from build123d import *

# Parameters (mm, degrees)
F0_R     = 9
F1_DEPTH = 19.3
F2_R     = 1
F3_R     = 4.68
F4_DEPTH = 10
F5_R     = 4
F6_DEPTH = 25


with BuildPart() as f1:
    # F0 (on Front) → F1 (new body)
    with BuildSketch(Plane.XZ):
        with BuildLine():
            ThreePointArc((-15.21127, 25.205598), (-18.278647, 23.530867), (-19.5, 20.256447))
            Line((-19.5, 20.256447), (-19.5, -22.20694))
            Line((-19.5, -22.20694), (-10.5, -22.20694))
            Line((-10.5, -22.20694), (-10.5, -20.20694))
            Line((-10.5, -20.20694), (10.5, -20.20694))
            Line((10.5, -20.20694), (10.5, -22.20694))
            Line((10.5, -22.20694), (19.5, -22.20694))
            Line((19.5, -22.20694), (19.5, 20.256447))
            ThreePointArc((19.5, 20.256447), (18.278647, 23.530867), (15.21127, 25.205598))
            ThreePointArc((15.21127, 25.205598), (0, 26.29306), (-15.21127, 25.205598))
        make_face()
        with Locations((0, 5.29306)):
            Circle(F0_R, mode=Mode.SUBTRACT)
    extrude(amount=F1_DEPTH)

    # F2
    f2_edges = [f1.edges().sort_by_distance(p)[0] for p in [
        (-10.5, -9.65, -20.20694),
        (10.5, -9.65, -20.20694),
    ]]
    fillet(f2_edges, radius=F2_R)

    # F3 (on Front) → F4 (join)
    with BuildSketch(Plane.XZ):
        with BuildLine():
            Line((34, 21.061159), (19.5, 21.061159))
            Line((19.5, 21.061159), (19.5, -4.20694))
            Line((19.5, -4.20694), (36.250328, -0.7062))
            ThreePointArc((36.250328, -0.7062), (44.941685, 11.192319), (34, 21.061159))
        make_face()
        with Locations((34, 10.061159)):
            Circle(F3_R, mode=Mode.SUBTRACT)
    extrude(amount=F4_DEPTH)

    # F5 (on face) → F6 (cut)
    with BuildSketch(Plane(origin=(0, 0, -20.20694), x_dir=(1, 0, 0), z_dir=(0, 0, -1))):
        with Locations((0, 9.65)):
            Circle(F5_R)
    extrude(amount=-F6_DEPTH, mode=Mode.SUBTRACT)


solid = f1.part
Here's how the part is built. I have some questions about the finished solid (model axes, mm). A direction names the side the tool comes from. Round coordinates to 2 decimals unless told otherwise and drop trailing zeros. Order: outer loops, then holes, each group sorted by start corner. A loop starts at its lowest first (then second) coordinate and runs counter-clockwise, first axis right, second up. Notation, with made-up numbers: (76.5, 50.25) -> (86.5, 50.25) arc R20 cw to (86.5, 70.25) -> close; hole circle Ø5 at (57, 82). An arc over 180 degrees is marked (long way). Return JSON: item names as keys, results as strings.
Q1. If we section it at D-D on y = -8.25: List the corners of the cut face in (x, z) for me.
Filled sheet:
{"outline": "(-19.5, -22.21) -> (-10.5, -22.21) -> (-10.5, -21.21) arc R1 cw to (-9.5, -20.21) -> (-3.75, -20.21) -> (-3.75, -2.89) arc R9 cw (long way) to (3.75, -2.89) -> (3.75, -20.21) -> (9.5, -20.21) arc R1 cw to (10.5, -21.21) -> (10.5, -22.21) -> (19.5, -22.21) -> (19.5, -4.21) -> (36.25, -0.71) arc R11 ccw to (34, 21.06) -> (19.5, 21.06) -> (19.5, 20.26) arc R5 ccw to (15.21, 25.21) arc R106.93 ccw to (-15.21, 25.21) arc R5 ccw to (-19.5, 20.26) -> close; hole circle Ø9.36 at (34, 10.06)"}
Q2. For pin 1 Ø8.5 at (x, z) = (34, 10.06) entering from -Y; pin 2 Ø8 at (y, z) = (-11, -13) entering from +X; pin 3 Ø0.9 at (y, z) = (-3.5, 21) entering from -X; pin 4 Ø3 at (x, y) = (27, -3) entering from +Z, each with a flat end and sliding along its axis, tell me the tip position at first contact or that it passes through.
Filled sheet:
{"pin 1": "passes through", "pin 2": "stops at x = 19.5", "pin 3": "stops at x = -19.49", "pin 4": "stops at z = 21.06"}
Q3. If we section it at B-B on z = 11: List the corners of the cut face in (x, y) for me, plus the area to 3 significant figures.
Filled sheet:
{"outline": "(-19.5, -19.3) -> (-6.96, -19.3) -> (-6.96, 0) -> (-19.5, 0) -> close; (6.96, -19.3) -> (19.5, -19.3) -> (19.5, -10) -> (29.42, -10) -> (29.42, 0) -> (6.96, 0) -> close; (38.58, -10) -> (44.96, -10) -> (44.96, 0) -> (38.58, 0) -> close", "area": "647 mm^2"}
Q4. Which directions (+Z, -Z, +X, -X, +Y, -Y) give clear straight access to the entire face, cutting with the end or side of a thin tool? Please do faces 4 (the flat face through (29, -10, 9)), 5 (the cylindrical face through (30.551, -4.93, 13.224)), 6 (the cylindrical face through (3.8, -10.9, -11.6)), 7 (the flat face through (19.5, -12, -6)).
Filled sheet:
{"face 4": "+Z, -Z, +X, -Y", "face 5": "+Y, -Y", "face 6": "-Z", "face 7": "-Z, +X, -Y"}
Q5. If we section it at A-A on x = 0: List the corners of the cut face in (y, z) for me.
Filled sheet:
{"outline": "(-19.3, -20.21) -> (-13.65, -20.21) -> (-13.65, -3.71) -> (-19.3, -3.71) -> close; (-19.3, 14.29) -> (0, 14.29) -> (0, 26.29) -> (-19.3, 26.29) -> close; (-5.65, -20.21) -> (0, -20.21) -> (0, -3.71) -> (-5.65, -3.71) -> close"}
Q6. I need wall thicknesses on line 1 along Y through (x, z) = (0, -11); line 2 along Z through (x, y) = (0, -5.25); line 3 along X through (y, z) = (-9.65, -15). Which ranges of each line are inside material? Lowest first, please. Write a range as from..to.
Filled sheet:
{"line 1": "y = -19.3..-13.65, -5.65..0", "line 2": "z = -20.21..-3.71, 14.29..26.29", "line 3": "x = -19.5..-4, 4..19.5"}
Q7. If we mould it in two halves opening along Z, with no side actions, what happens to faces 1 (the cylindrical face through (4.84, -9.51, 12.88)), 2 (the flat face through (-4.4, -9.5, -20.207)), 3 (the flat face through (27, -5, 21.061))? For each: released by +Z, released by -Z, zero draft, split by the parting line, or undercut.
Filled sheet:
{"face 1": "undercut", "face 2": "released by -Z", "face 3": "released by +Z"}
Q8. If we section it at C-C on z = -9.5: List the corners of the cut face in (x, y) for me, plus the area to 3 significant figures.
Filled sheet:
{"outline": "(-19.5, -19.3) -> (19.5, -19.3) -> (19.5, 0) -> (-19.5, 0) -> close; hole circle Ø8 at (0, -9.65)", "area": "702 mm^2"}
